from build123d import *

# Parameters (mm, degrees)
F0_R     = 12.5
F0_R_2   = 4
F1_DEPTH = 11
F2_DEPTH = 15
F3_DEPTH = 9.5
F5_R     = 3
F6_SIZE  = 1.99999


# Not quite as in the source:
# - a fillet or chamfer that OpenCascade refuses, or shapes differently, is made with other operations: its cross-section is extruded or revolved along the edge and cut away or added
# - a fillet or chamfer is up to 0.001 mm smaller than in the source, because OpenCascade refuses the exact size


with BuildPart() as f1:
    # F0 (on Front) → F1 (new body)
    with BuildSketch(Plane.XZ):
        with BuildLine():
            Line((15.5, -22.5), (22.5, -22.5))
            Line((22.5, -22.5), (22.5, -15.5))
            Line((22.5, -15.5), (17.5, -15.5))
            ThreePointArc((17.5, -15.5), (16.9142135624, -16.9142135624), (15.5, -17.5))
            Line((15.5, -17.5), (15.5, -22.5))
        make_face()
        with BuildLine():
            Line((-15.5, -22.5), (15.5, -22.5))
            Line((15.5, -22.5), (15.5, -17.5))
            ThreePointArc((15.5, -17.5), (14.0857864376, -14.0857864376), (17.5, -15.5))
            Line((17.5, -15.5), (22.5, -15.5))
            Line((22.5, -15.5), (22.5, 15.5))
            Line((22.5, 15.5), (17.5, 15.5))
            ThreePointArc((17.5, 15.5), (14.0857864376, 14.0857864376), (15.5, 17.5))
            Line((15.5, 17.5), (15.5, 22.5))
            Line((15.5, 22.5), (-15.5, 22.5))
            Line((-15.5, 22.5), (-15.5, 17.5))
            ThreePointArc((-15.5, 17.5), (-14.0857864376, 16.9142135624), (-13.5, 15.5))
            ThreePointArc((-13.5, 15.5), (-15.5, 13.5), (-17.5, 15.5))
            Line((-17.5, 15.5), (-22.5, 15.5))
            Line((-22.5, 15.5), (-22.5, -15.5))
            Line((-22.5, -15.5), (-17.5, -15.5))
            ThreePointArc((-17.5, -15.5), (-15.5, -13.5), (-13.5, -15.5))
            ThreePointArc((-13.5, -15.5), (-14.0857864376, -16.9142135624), (-15.5, -17.5))
            Line((-15.5, -17.5), (-15.5, -22.5))
        make_face()
        Circle(F0_R, mode=Mode.SUBTRACT)
        with BuildLine():
            Line((-22.5, -22.5), (-15.5, -22.5))
            Line((-15.5, -22.5), (-15.5, -17.5))
            ThreePointArc((-15.5, -17.5), (-16.9142135624, -16.9142135624), (-17.5, -15.5))
            Line((-17.5, -15.5), (-22.5, -15.5))
            Line((-22.5, -15.5), (-22.5, -22.5))
        make_face()
        with BuildLine():
            Line((17.5, 15.5), (22.5, 15.5))
            Line((22.5, 15.5), (22.5, 22.5))
            Line((22.5, 22.5), (15.5, 22.5))
            Line((15.5, 22.5), (15.5, 17.5))
            ThreePointArc((15.5, 17.5), (16.9142135624, 16.9142135624), (17.5, 15.5))
        make_face()
        with BuildLine():
            Line((-22.5, 22.5), (-22.5, 15.5))
            Line((-22.5, 15.5), (-17.5, 15.5))
            ThreePointArc((-17.5, 15.5), (-16.9142135624, 16.9142135624), (-15.5, 17.5))
            Line((-15.5, 17.5), (-15.5, 22.5))
            Line((-15.5, 22.5), (-22.5, 22.5))
        make_face()
        Circle(F0_R)
        Polygon((8.0829037687, 0), (4.0414518843, -7), (-4.0414518843, -7), (-8.0829037687, 0), (-4.0414518843, 7), (4.0414518843, 7), align=None, mode=Mode.SUBTRACT)
        Polygon((-4.0414518843, -7), (4.0414518843, -7), (8.0829037687, 0), (4.0414518843, 7), (-4.0414518843, 7), (-8.0829037687, 0), align=None)
        Circle(F0_R_2, mode=Mode.SUBTRACT)
    extrude(amount=-F1_DEPTH)

    # F0 (on Front) → F2 (join)
    with BuildSketch(Plane.XZ):
        Circle(F0_R)
        Polygon((8.0829037687, 0), (4.0414518843, -7), (-4.0414518843, -7), (-8.0829037687, 0), (-4.0414518843, 7), (4.0414518843, 7), align=None, mode=Mode.SUBTRACT)
        Polygon((-4.0414518843, -7), (4.0414518843, -7), (8.0829037687, 0), (4.0414518843, 7), (-4.0414518843, 7), (-8.0829037687, 0), align=None)
        Circle(F0_R_2, mode=Mode.SUBTRACT)
    extrude(amount=-F2_DEPTH)

    # F0 (on Front) → F3 (cut)
    with BuildSketch(Plane.XZ):
        Polygon((-4.0414518843, -7), (4.0414518843, -7), (8.0829037687, 0), (4.0414518843, 7), (-4.0414518843, 7), (-8.0829037687, 0), align=None)
        Circle(F0_R_2, mode=Mode.SUBTRACT)
    extrude(amount=-F3_DEPTH, mode=Mode.SUBTRACT)

    # F4: fillet of radius 5 on 1 edges, made by hand

    # F4_s1 → F4_t2 (revolve)
    with BuildSketch(Plane.XY):
        with BuildLine():
            ThreePointArc((17.3989794856, 11), (14.2367018254, 12.1270166538), (12.5, 15))
            Line((12.5, 15), (12.5, 11))
            Line((12.5, 11), (17.3989794856, 11))
        make_face()
    revolve(axis=Axis((0, 11, 0), (0, -1, 0)))

    # F5
    f5_edges = [f1.edges().sort_by_distance(p)[0] for p in [
        (-12.5, 15, 0),
        (0, 11, -22.5),
        (-22.5, 11, 0),
        (-22.5, 5.5, -22.5),
        (-22.5, 5.5, 22.5),
        (0, 11, 22.5),
        (22.5, 5.5, 22.5),
        (22.5, 11, 0),
        (22.5, 5.5, -22.5),
    ]]
    fillet(f5_edges, radius=F5_R)

    # F6 (size 2 in the source; OpenCascade refuses exactly that, so slightly less here)
    f6_edges = [f1.edges().sort_by_distance(p)[0] for p in [
        (-13.5, 11, 15.5),
        (-15.5, 11, -13.5),
        (15.5, 11, -13.5),
        (15.5, 11, 13.5),
    ]]
    chamfer(f6_edges, length=F6_SIZE)


solid = f1.part
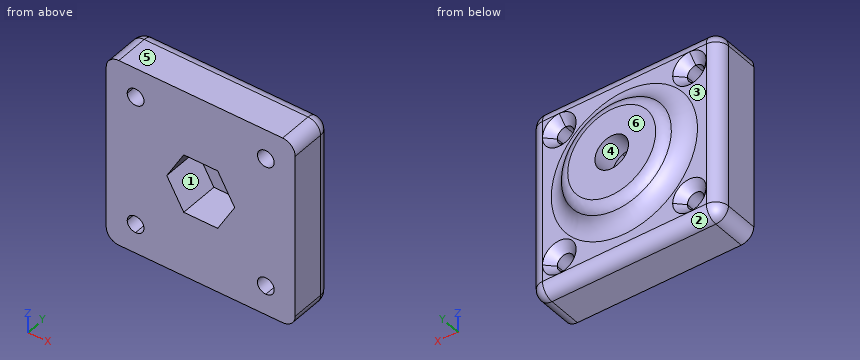
Can you work these out from the model? Positions are in its coordinate system, mm. Face numbers are marked on the shaded views. A direction names the side the tool comes from. Coordinates: 2 decimals unless noted, no trailing zeros. Write each loop counter-clockwise with the first axis right and the second up, starting at its lowest first coordinate (ties: lowest second). Pieces come first, ordered by that corner, then holes.
Q1. Please list where these lines run through material, in increasing order: L1, parallel to X at y = 7, z = 15.5; L2, parallel to Z at x = 3, y = 8; L3, parallel to Z at x = 16.5, y = 8.
Results found:
L1: x = -22.5 to -17.5, -13.5 to 13.5, 17.5 to 22.5
L2: z = -22.5 to -7, 7 to 22.5
L3: z = -22.5 to -17.23, -13.77 to 13.77, 17.23 to 22.5
Q2. Imagine slicing it at C-C, the plane y = 12.25. List the corners of the cut face in (x, z) for me, plus the area to 3 significant figures.
Results found:
outline: circle Ø28.18 at (0, 0); hole circle Ø8 at (0, 0)
area: 574 mm2
Q3. Which directions (+Z, -Z, +X, -X, +Y, -Y) give clear straight access to the entire face, cutting with the end or side of a thin tool? Please do the marked faces 1, 2 and 3.
Results found:
face 1: -Y
face 2: -Z, +X, -X, +Y
face 3: +Y
Q4. For P1, Ø12, axis at x = 11.5, z = 18, coming from the +Y side; P2, Ø3, axis at x = 3.5, z = 18, coming from the -Y side; P3, Ø5, axis at x = 0, z = 0, coming from the -Y side; P4, Ø1.5, axis at x = 8.5, y = 10.5, coming from the +Z side, each with a flat end and sliding along its axis, tell me the tip position at first contact or that it passes through.
Results found:
P1: stops at y = 11.43
P2: stops at y = 0
P3: passes through
P4: stops at z = 21.94
Q5. If we mould it in two halves opening along Z, with no side actions, what happens to the marked faces 4, 5 and 6? For each: +Z half, -Z half, draft (parallel to the pull), parting line (faces both ways), or undercut.
Results found:
face 4: undercut
face 5: +Z half
face 6: draft
Q6. Imagine slicing it at B-B, the plane z = 14.5. Count the separate pieces of the cut face and the enclosed holes in it, plus the area to 3 significant figures.
Results found:
separate pieces: 3
enclosed holes: 0
area: 415 mm2
Q7. Imagine slicing it at A-A, the plane y = 3. List the corners of the cut face in (x, z) for me, plus the area to 3 significant figures.
Results found:
outline: (-22.5, -19.5) arc R3 ccw to (-19.5, -22.5) - (19.5, -22.5) arc R3 ccw to (22.5, -19.5) - (22.5, 19.5) arc R3 ccw to (19.5, 22.5) - (-19.5, 22.5) arc R3 ccw to (-22.5, 19.5) - close; hole circle Ø4 at (-15.5, -15.5); hole circle Ø4 at (-15.5, 15.5); hole (-8.08, 0) - (-4.04, -7) - (4.04, -7) - (8.08, 0) - (4.04, 7) - (-4.04, 7) - close; hole circle Ø4 at (15.5, -15.5); hole circle Ø4 at (15.5, 15.5)
area: 1,800 mm2
